Input: part model. Units: mm. Frame: model coordinates. Face numbers are marked on the shaded views. Coordinates: 2 decimals unless noted, no trailing zeros. Write each loop counter-clockwise with the first axis right and the second up, starting at its lowest first coordinate (ties: lowest second). Pieces come first, ordered by that corner, then holes. Notation, with made-up numbers: (-7, -5) -> (44, -5) arc R20 ccw to (44, 2) -> close; hole circle Ø3 at (71, 45.5). An arc over 180 degrees is marked (long way). Use one line per item in the form item = value. Start each with the question number.
(1) Cut plane C-C on z = -13.5. Return the cut outline in (x, y).
(2) Cut plane B-B on y = -33. Return the cut outline in (x, z).
(3) Ray query, line 1 along Y through (x, z) = (1.25, -20.5); line 2 along Z through (x, y) = (6.5, -24.5) (1 decimal); line 3 along Y through (x, z) = (7, -23). Return the intervals inside material, ascending.
(4) Pull-direction query (Y, two-part tool) for the marked faces 1, 2 and 3; classes: released by +Y, released by -Y, zero draft, split by the parting line, or undercut.
(5) First-contact query: pin 1 (18 mm diameter, centred on y = -25, z = -20, fed in from +X); pin 2 (5 mm diameter, centred on y = -23.5, z = -73, fed in from -X); pin 3 (3 mm diameter, centred on x = 6.5, y = -21.5, fed in from +Z); pin 4 (2 mm diameter, centred on x = 8, y = -23.5, fed in from +Z) (3 decimals). Flat tips, straight axial feed; report the tip coordinate or a pass-through.
(6) Cut plane D-D on y = -9. Return the cut outline in (x, z).
(7) Cut plane A-A on x = 9. Return the cut outline in (y, z).
```python
from build123d import *

# Parameters (mm, degrees)
SKETCH1_R           = 10
BOSS_EXTRUDE1_DEPTH = 10
FILLET1_R           = 10


with BuildPart() as part:
    # Sketch1 → Boss-Extrude1 (new body)
    with BuildSketch(Plane(origin=(0, 0, 0), x_dir=(0, 0, -1), z_dir=(1, 0, 0))):
        with BuildLine():
            Line((20, 0), (100, 0))
            Line((100, 0), (100, -50))
            Line((100, -50), (20, -50))
            ThreePointArc((20, -50), (-5, -25), (20, 0))
        make_face()
        with Locations((20, -25)):
            Circle(SKETCH1_R, mode=Mode.SUBTRACT)
    extrude(amount=BOSS_EXTRUDE1_DEPTH)

    # Fillet1
    fillet1_edges = [part.edges().sort_by_distance(p)[0] for p in [
        (5, -50, -100),
        (5, 0, -100),
    ]]
    fillet(fillet1_edges, radius=FILLET1_R)


solid = part.part
```
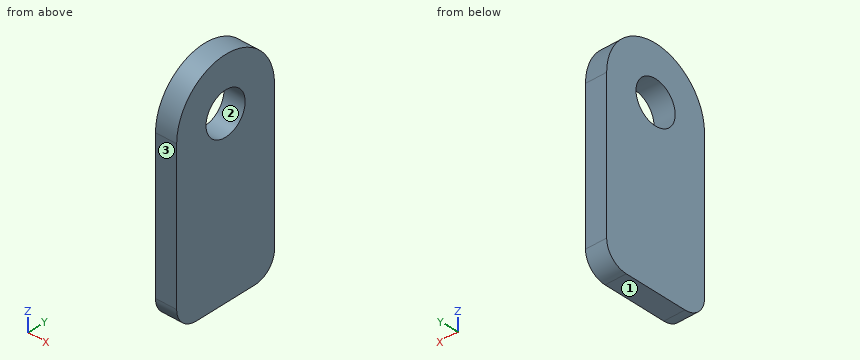
Values:
q1.outline = (0, -49.14) -> (10, -49.14) -> (10, -32.6) -> (0, -32.6) -> close; (0, -17.4) -> (10, -17.4) -> (10, -0.86) -> (0, -0.86) -> close
q2.outline = (0, -100) -> (10, -100) -> (10, -26) -> (0, -26) -> close; (0, -14) -> (10, -14) -> (10, 3.69) -> (0, 3.69) -> close
q3.line_1 = -50 to -34.99, -15.01 to 0
q3.line_2 = -100 to -30, -10 to 5
q3.line_3 = -50 to -34.54, -15.46 to 0
q4.face_1 = zero draft
q4.face_2 = undercut
q4.face_3 = released by -Y
q5.pin_1 = through
q5.pin_2 = 0
q5.pin_3 = 4.92
q5.pin_4 = 4.995
q6.outline = (0, -99.95) -> (10, -99.95) -> (10, -0.79) -> (0, -0.79) -> close
q7.outline = (-50, -90) arc R10 ccw to (-40, -100) -> (-10, -100) arc R10 ccw to (0, -90) -> (0, -20) arc R25 ccw to (-50, -20) -> close; hole circle Ø20 at (-25, -20)
